```python
from build123d import *

# Parameters (mm, degrees)
SKETCH1_W           = 93
SKETCH1_H           = 66.8
BOSS_EXTRUDE1_DEPTH = 1.25
FILLET1_R           = 2
SKETCH2_W           = 93
SKETCH2_H           = 66.8
CUT_EXTRUDE1_DEPTH  = 1
SKETCH3_R           = 1
CUT_EXTRUDE2_DEPTH  = 0.75
SKETCH4_R           = 1.45
BOSS_EXTRUDE2_DEPTH = 5
SKETCH5_R           = 2.5
BOSS_EXTRUDE3_DEPTH = 1.8


with BuildPart() as part:
    # Sketch1 → Boss-Extrude1 (new, symmetric)
    with BuildSketch(Plane(origin=(0, 0, 0), x_dir=(1, 0, 0), z_dir=(0, 1, 0))):
        Rectangle(SKETCH1_W, SKETCH1_H)
    extrude(amount=BOSS_EXTRUDE1_DEPTH, both=True)

    # Fillet1
    fillet1_edges = [part.edges().sort_by_distance(p)[0] for p in [
        (0, 1.25, -33.4),
        (-46.5, 1.25, 0),
        (0, 1.25, 33.4),
    ]]
    fillet(fillet1_edges, radius=FILLET1_R)

    # Sketch2 → Cut-Extrude1 (cut)
    with BuildSketch(Plane.XZ.offset(1.25)):
        Rectangle(SKETCH2_W, SKETCH2_H)
    extrude(amount=-CUT_EXTRUDE1_DEPTH, mode=Mode.SUBTRACT)

    # Sketch3 → Cut-Extrude2 (cut)
    with BuildSketch(Plane.XZ.offset(0.25)):
        with Locations(Location((-43.5, 30.4, 0), (0, 0, 270))):
            Circle(SKETCH3_R)
        with Locations(Location((43.5, 30.4, 0), (0, 0, 270))):
            Circle(SKETCH3_R)
        with Locations(Location((43.5, -30.4, 0), (0, 0, 270))):
            Circle(SKETCH3_R)
        with Locations(Location((-43.5, -30.4, 0), (0, 0, 270))):
            Circle(SKETCH3_R)
    extrude(amount=-CUT_EXTRUDE2_DEPTH, mode=Mode.SUBTRACT)

    # Sketch4 → Boss-Extrude2 (add)
    with BuildSketch(Plane.XZ.offset(0.25)):
        with Locations(Location((-37.55, 26.486491673, 0), (0, 0, 270))):
            Circle(SKETCH4_R)
        with Locations(Location((17.55, 26.486491673, 0), (0, 0, 270))):
            Circle(SKETCH4_R)
        with Locations(Location((17.55, -19.613508327, 0), (0, 0, 270))):
            Circle(SKETCH4_R)
        with Locations(Location((-37.55, -19.613508327, 0), (0, 0, 270))):
            Circle(SKETCH4_R)
    extrude(amount=BOSS_EXTRUDE2_DEPTH)

    # Sketch5 → Boss-Extrude3 (add)
    with BuildSketch(Plane.XZ.offset(0.25)):
        with Locations(Location((-37.55, 26.486491673, 0), (0, 0, 270))):
            Circle(SKETCH5_R)
        with Locations(Location((17.55, 26.486491673, 0), (0, 0, 270))):
            Circle(SKETCH5_R)
        with Locations(Location((17.55, -19.613508327, 0), (0, 0, 270))):
            Circle(SKETCH5_R)
        with Locations(Location((-37.55, -19.613508327, 0), (0, 0, 270))):
            Circle(SKETCH5_R)
    extrude(amount=BOSS_EXTRUDE3_DEPTH)


solid = part.part
```
For this review, take the finished solid that the model builds, in its own axes (mm). A direction names the side the tool comes from. Coordinates: 2 decimals unless noted, no trailing zeros. Order: outer loops, then holes, each group sorted by start corner. A loop starts at its lowest first (then second) coordinate and runs counter-clockwise, first axis right, second up. Notation, with made-up numbers: (-37, -39) - (4, -39) arc R26 cw to (4, -25) - close; hole circle Ø5 at (76, 80.5). An arc over 180 degrees is marked (long way). Answer as a JSON object with one key per item and string values. Group by question number.
1. We need section C-C on x = -37.55. State the section outline as (y, z) points, then the cut area to 3 significant figures.
2. We need section B-B on y = -3.75. State the section outline as (x, z) points, then the cut area to 3 significant figures.
3. Clearance check with flat-ended pins moving along their axes: P1, Ø2, axis at x = 43, z = -30.5, coming from the -Y side; P2, Ø1.2, axis at x = 43.5, z = -30.4, coming from the -Y side. State where each tip first meets the part, or that it passes through.
4. For faces 3 (the flat face through (16, -2.05, 25)), 4 (the flat face through (-38, -5.25, -20)), list the 3-axis set-ups (+Z, -Z, +X, -X, +Y, -Y) from which the entire face can be reached by the end or side of a thin tool; tool diameter is ignored.
5. We need section D-D on x = 43.5. State the section outline as (y, z) points, then the cut area to 3 significant figures.
6. The part is to be moulded in two halves that separate along Z. For faces 1 (the flat face through (0, 1.25, 0)), 2 (the cylindrical face through (16.59, -1.14, -21.92)), say which applies: pulls with the +Z half, pulls with the -Z half, needs draft (parallel to the pull), parting line crosses it, or undercut.
7. For probe 1 along X at (y, z) = (0.1, -30.4); probe 2 along Y at (x, z) = (23, -13); probe 3 along Z at (x, y) = (16, -0.75), list the stretches that pass through material, from the lowest coordinate up.
8. We need section A-A on z = -30.4. State the section outline as (x, y) points.
Final values:
{
 "1": {"outline": "(-5.25, -21.06) - (-2.05, -21.06) - (-2.05, -22.11) - (-0.25, -22.11) - (-0.25, -33.34) arc R2 ccw to (1.25, -31.4) - (1.25, 31.4) arc R2 ccw to (-0.25, 33.34) - (-0.25, 28.99) - (-2.05, 28.99) - (-2.05, 27.94) - (-5.25, 27.94) - (-5.25, 25.04) - (-2.05, 25.04) - (-2.05, 23.99) - (-0.25, 23.99) - (-0.25, -17.11) - (-2.05, -17.11) - (-2.05, -18.16) - (-5.25, -18.16) - close", "area": "135 mm²"},
 "2": {"outline": "circle Ø2.9 at (-37.55, -19.61); circle Ø2.9 at (-37.55, 26.49); circle Ø2.9 at (17.55, -19.61); circle Ø2.9 at (17.55, 26.49)", "area": "26.4 mm²"},
 "3": {"P1": "y = -0.25", "P2": "y = 0.5"},
 "4": {"face 3": "-Y", "face 4": "+Z, -Z, +X, -X, -Y"},
 "5": {"outline": "(-0.25, -33.34) arc R2 ccw to (1.25, -31.4) - (1.25, 31.4) arc R2 ccw to (-0.25, 33.34) - (-0.25, 31.4) - (0.5, 31.4) - (0.5, 29.4) - (-0.25, 29.4) - (-0.25, -29.4) - (0.5, -29.4) - (0.5, -31.4) - (-0.25, -31.4) - close", "area": "95.5 mm²"},
 "6": {"face 1": "needs draft", "face 2": "undercut"},
 "7": {"probe 1": "-46.31 to -44.5, -42.5 to 42.5, 44.5 to 46.5", "probe 2": "-0.25 to 1.25", "probe 3": "-21.58 to -17.65, 24.52 to 28.45"},
 "8": {"outline": "(-46.44, -0.25) - (-44.5, -0.25) - (-44.5, 0.5) - (-42.5, 0.5) - (-42.5, -0.25) - (42.5, -0.25) - (42.5, 0.5) - (44.5, 0.5) - (44.5, -0.25) - (46.5, -0.25) - (46.5, 1.25) - (-44.5, 1.25) arc R2 ccw to start"}
}
